Could you check a few things on this drawing? It's one solid part, dimensions in mm from its lowest x, y, z. Round coordinates to 2 decimals unless told otherwise and drop trailing zeros. Loops run counter-clockwise (first coordinate to the right, second up) from the corner with the lowest first, then second, coordinate; pieces in that order, holes last. Notation, with made-up numbers: (-32, -7) -> (5, -7) arc R20 ccw to (5, 13) -> close; hole circle Ø11 at (38.25, 84). An arc over 180 degrees is marked (long way). Use one line per item in the form item = value. Start each with the question number.
Item 1: If we section it at B-B (z = 87.5): Write out the boundary of the cut face in (x, y).
Item 2: If we section it at A-A (y = 1.35): Write out the boundary of the cut face in (x, z).
Item 3: If we section it at C-C (x = 35): Write out the boundary of the cut face in (y, z), then the cut area to 3 significant figures.
Item 4: Thinking about a two-plate mould opening in Z: for the marked faces 1 and 2, which applies, released by +Z, released by -Z, zero draft, split by the parting line, or undercut?
Item 5: If I drill on L1, parallel to X at y = 2, z = 22.5; L2, parallel to Z at x = 82, y = 1.85; L3, parallel to Y at x = 114.5, z = 29, over which ranges is the centre line in solid material (lowest first)? Write a range as [from, to].
Item 6: I'm going to push flat-ended pins straight in: pin 1 Ø12 at (x, z) = (134, 96) entering from -Y; pin 2 Ø1.5 at (x, y) = (55, 1) entering from +Z; pin 3 Ø1.5 at (y, z) = (1.5, 38.5) entering from -X; pin 4 Ø3.5 at (x, y) = (54, 2) entering from -Z. Where does each tip first touch, or does it pass through?
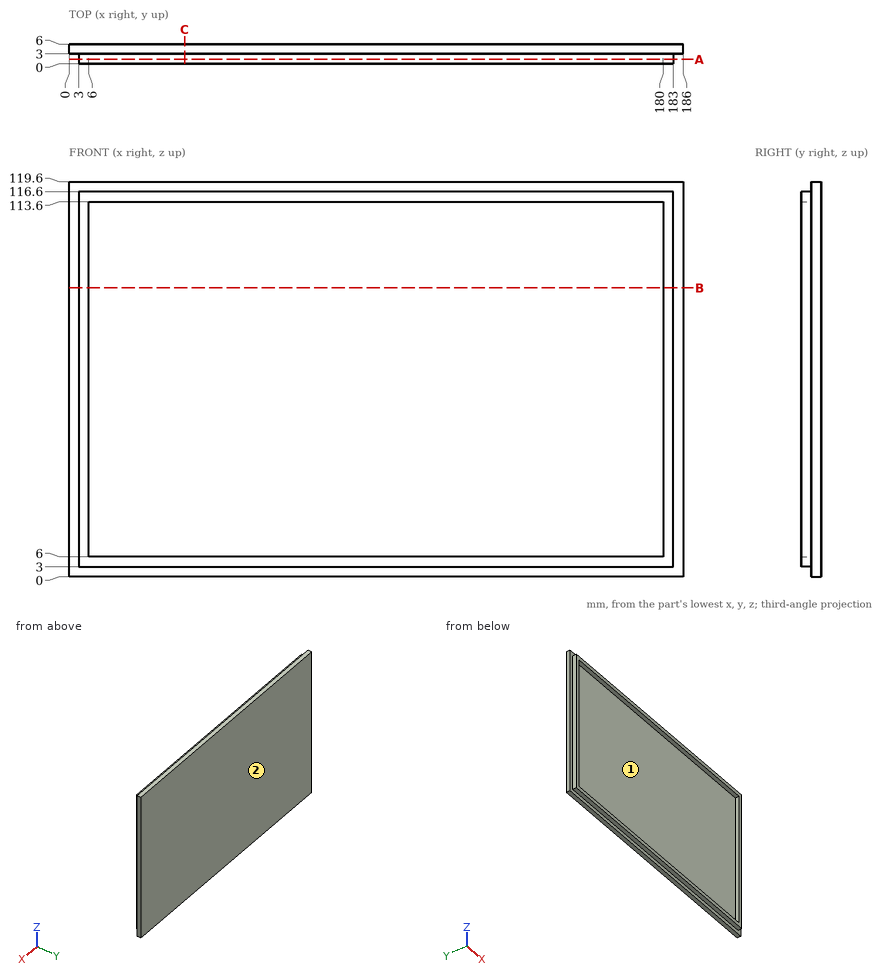
Values found:
q1.outline = (0, 3) -> (3, 3) -> (3, 0) -> (6, 0) -> (6, 3) -> (180, 3) -> (180, 0) -> (183, 0) -> (183, 3) -> (186, 3) -> (186, 6) -> (0, 6) -> close
q2.outline = (3, 3) -> (183, 3) -> (183, 116.6) -> (3, 116.6) -> close; hole (6, 6) -> (180, 6) -> (180, 113.6) -> (6, 113.6) -> close
q3.outline = (0, 3) -> (3, 3) -> (3, 0) -> (6, 0) -> (6, 119.6) -> (3, 119.6) -> (3, 116.6) -> (0, 116.6) -> (0, 113.6) -> (3, 113.6) -> (3, 6) -> (0, 6) -> close
q3.area = 377 mm2
q4.face_1 = undercut
q4.face_2 = zero draft
q5.L1 = [3, 6], [180, 183]
q5.L2 = [3, 6], [113.6, 116.6]
q5.L3 = [3, 6]
q6.pin_1 = 3
q6.pin_2 = 116.6
q6.pin_3 = 3
q6.pin_4 = 0
